Verification items for the finished model (mm, model axes). Face numbers are marked on the shaded views. Coordinates: 2 decimals unless noted, no trailing zeros. Order: outer loops, then holes, each group sorted by start corner. A loop starts at its lowest first (then second) coordinate and runs counter-clockwise, first axis right, second up. Notation, with made-up numbers: M -27,25 L -14,25 A25 ccw -14,48 Z; hole C -3.5,38 d4. An arc over 180 degrees is marked long. Return JSON: item names as keys, results as strings.
```python
from build123d import *

# Parameters (mm, degrees)
F0_W     = 80
F0_H     = 80
F1_DEPTH = 40
F2_R     = 5
F3_R     = 15
F4_DEPTH = 40.001


with BuildPart() as f1:
    # F0 (on Top) → F1 (new body, symmetric)
    with BuildSketch(Plane.XY):
        Rectangle(F0_W, F0_H)
    extrude(amount=F1_DEPTH, both=True)

    # F2
    f2_edges = [f1.edges().sort_by_distance(p)[0] for p in [
        (0, 40, 40),
        (-40, 0, 40),
        (0, -40, 40),
        (40, 0, 40),
        (40, -40, 0),
        (40, 40, 0),
        (40, 0, -40),
        (0, -40, -40),
        (-40, -40, 0),
        (-40, 0, -40),
        (0, 40, -40),
        (-40, 40, 0),
    ]]
    fillet(f2_edges, radius=F2_R)

    # F3 (on Top) → F4 (cut, through all)
    with BuildSketch(Plane.XY):
        Circle(F3_R)
    extrude(amount=F4_DEPTH, mode=Mode.SUBTRACT)


solid = f1.part
```
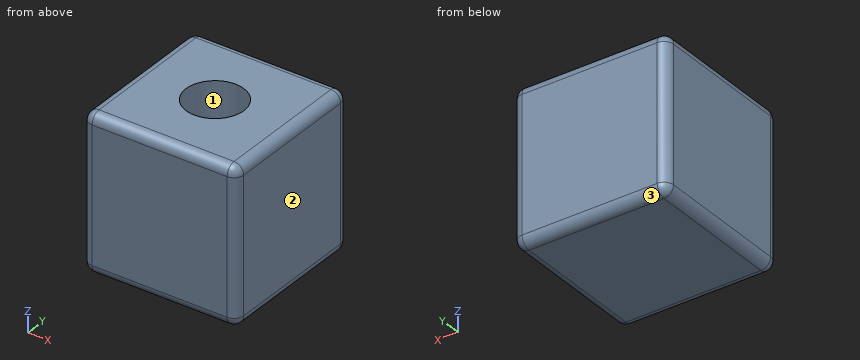
Q1. Cross-section at A-A, the plane z = 14. Record the boundary of the cut face in (x, y).
Values:
{"outline": "M -40,-35 A5 ccw -35,-40 L 35,-40 A5 ccw 40,-35 L 40,35 A5 ccw 35,40 L -35,40 A5 ccw -40,35 Z; hole C 0,0 d30"}
Q2. Material ranges on line 1 along Y through (x, z) = (0, 11); line 2 along Z through (x, y) = (-9.5, 2.5), recorded low to high.
Values:
{"line 1": "-40 to -15, 15 to 40", "line 2": "-40 to 0"}
Q3. Cross-section at C-C, the plane x = 0. Record the boundary of the cut face in (y, z), and give its area (3 significant figures).
Values:
{"outline": "M -40,-35 A5 ccw -35,-40 L 35,-40 A5 ccw 40,-35 L 40,35 A5 ccw 35,40 L 15,40 L 15,0 L -15,0 L -15,40 L -35,40 A5 ccw -40,35 Z", "area": "5,180 mm^2"}
Q4. Cross-section at B-B, the plane y = 12. Record the boundary of the cut face in (x, z).
Values:
{"outline": "M -40,-35 A5 ccw -35,-40 L 35,-40 A5 ccw 40,-35 L 40,35 A5 ccw 35,40 L 9,40 L 9,0 L -9,0 L -9,40 L -35,40 A5 ccw -40,35 Z"}
Q5. Go/stop test with a flat-tipped pin: pin 1 (8 mm diameter, centred on x = 6.5, y = -8.5, fed in from +Z). Record where the tip stops, or that it passes through.
Values:
{"pin 1": "z = 0"}
Q6. Draft check along Y on the marked faces 1, 2 and 3. Enter one of: pulls with the +Y half, pulls with the -Y half, needs draft (parallel to the pull), parting line crosses it, or undercut.
Values:
{"face 1": "undercut", "face 2": "needs draft", "face 3": "pulls with the +Y half"}
